For this review, take the finished solid that the model builds, in its own axes (mm). Face numbers are marked on the shaded views. A direction names the side the tool comes from. Coordinates: 2 decimals unless noted, no trailing zeros. Write each loop counter-clockwise with the first axis right and the second up, starting at its lowest first coordinate (ties: lowest second). Pieces come first, ordered by that corner, then holes. Notation, with made-up numbers: M -5,-1.5 L 24,-1.5 A17 cw 24,11.5 Z; hole C -28,-30.5 d4. An arc over 180 degrees is marked long. One line per question, with ' | ' between items.
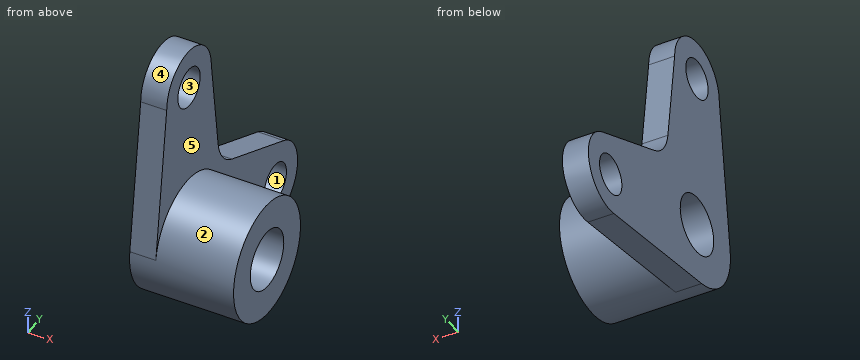
from build123d import *

# Parameters (mm, degrees)
SKETCH1_R           = 15
BOSS_EXTRUDE1_DEPTH = 20
SKETCH1_3_R         = 45
SKETCH1_3_R_2       = 22.5
BOSS_EXTRUDE2_DEPTH = 80


with BuildPart() as part:
    # Sketch1 → Boss-Extrude1 (new body)
    with BuildSketch(Plane.YZ):
        with BuildLine():
            ThreePointArc((30, 120), (0, 150), (-30, 120))
            Line((-30, 120), (-44.635477489, 5.716130628))
            ThreePointArc((-44.635477489, 5.716130628), (2.863870895, 44.908776909), (45, 0))
            ThreePointArc((45, 0), (29.576190824, -33.915320083), (-6.122174948, -44.581599051))
            Line((-6.122174948, -44.581599051), (111.829649189, -60.779351446))
            ThreePointArc((111.829649189, -60.779351446), (144.888873943, -38.822856765), (127.236992817, -3.278362217))
            Line((127.236992817, -3.278362217), (57.508255637, 25.150091561))
            ThreePointArc((57.508255637, 25.150091561), (45.052202352, 34.642888154), (39.077164307, 49.119261005))
            Line((39.077164307, 49.119261005), (30, 120))
        make_face()
        with Locations(Location((115.911099155, -31.058285412, 0), (0, 0, 270))):
            Circle(SKETCH1_R, mode=Mode.SUBTRACT)
        with Locations(Location((0, 120, 0), (0, 0, 270))):
            Circle(SKETCH1_R, mode=Mode.SUBTRACT)
    extrude(amount=BOSS_EXTRUDE1_DEPTH)

    # Sketch1_3 → Boss-Extrude2 (add)
    with BuildSketch(Plane.YZ):
        with Locations(Location((0, 0, 0), (0, 0, 172.702280721))):
            Circle(SKETCH1_3_R)
        with Locations(Location((0, 0, 0), (0, 0, 270))):
            Circle(SKETCH1_3_R_2, mode=Mode.SUBTRACT)
    extrude(amount=BOSS_EXTRUDE2_DEPTH)


solid = part.part
1) We need section D-D on x = 69.5. State the section outline as (y, z) points.
Responses:
outline: C 0,0 d90; hole C 0,0 d45
2) The part is to be moulded in two halves that separate along Z. For the marked faces 3, 4 and 5, say which applies: +Z half, -Z half, draft (parallel to the pull), parting line (faces both ways), or undercut.
Responses:
face 3: undercut | face 4: +Z half | face 5: draft
3) To check wall thickness, follow line 1 along Y through (x, z) = (51, 0); line 2 along X through (y, z) = (97, -2); line 3 along Z through (x, y) = (21.5, 17.5). State the ranges of each line that lie inside material, in increasing order. Write a range as [from, to].
Responses:
line 1: [-45, -22.5], [22.5, 45] | line 2: [0, 20] | line 3: [-41.46, -14.14], [14.14, 41.46]
4) Insertion check: pin 1 Ø10 at (x, y) = (23.5, 24.5) entering from -Z; pin 2 Ø5 at (x, z) = (8, -30) entering from -Y; pin 3 Ø10 at (y, z) = (38, 51) entering from -X; pin 4 Ø5 at (x, y) = (16.5, 118.5) entering from +Z. Each pin has a flat end and moves straight along its axis. Give the tip position at first contact, or say it passes through.
Responses:
pin 1: z = -49.28 | pin 2: y = -35.62 | pin 3: x = 0 | pin 4: z = 1.3
5) Machinability: for the marked faces 1 and 2, which of the approach directions +Z, -Z, +X, -X, +Y, -Y give a long, thin tool a straight path to every point of the face, cutting with its end or side? Answer none if there is none.
Responses:
face 1: +X, -X | face 2: +X
6) We need section C-C on x = 13.5. State the section outline as (y, z) points, then the cut area to 3 significant figures.
Responses:
outline: M -44.64,5.72 A45 ccw -6.12,-44.58 L 111.83,-60.78 A30 ccw 127.24,-3.28 L 57.51,25.15 A30 cw 39.08,49.12 L 30,120 A30 ccw -30,120 Z; hole C 0,0 d45; hole C 0,120 d30; hole C 115.91,-31.06 d30 | area: 17,900 mm^2
7) We need section A-A on y = 0. State the section outline as (x, z) points, then the cut area to 3 significant figures.
Responses:
outline: M 0,-45.42 L 20,-45.42 L 20,-45 L 80,-45 L 80,-22.5 L 0,-22.5 Z; M 0,22.5 L 80,22.5 L 80,45 L 20,45 L 20,105 L 0,105 Z; M 0,135 L 20,135 L 20,150 L 0,150 Z | area: 5,110 mm^2
8) We need section B-B on z = 0. State the section outline as (x, y) points, then the cut area to 3 significant figures.
Responses:
outline: M 0,-45 L 80,-45 L 80,-22.5 L 0,-22.5 Z; M 0,22.5 L 80,22.5 L 80,45 L 20,45 L 20,119.2 L 0,119.2 Z | area: 5,080 mm^2
